Build history of the part. All positions in model axes, mm. A direction names the side the tool comes from. Round coordinates to 2 decimals unless told otherwise and drop trailing zeros. Write each loop counter-clockwise with the first axis right and the second up, starting at its lowest first coordinate (ties: lowest second). Pieces come first, ordered by that corner, then holes. Notation, with made-up numbers: (52, 9) - (92, 9) arc R37 ccw to (92, 47) - close; hole circle Ø3 at (-38, 4.5). An arc over 180 degrees is marked (long way). Write each question's results on one line, items separated by ' | '.
from build123d import *

# Parameters (mm, degrees)
SKETCH1_W           = 35
SKETCH1_H           = 37
SKETCH1_R           = 1.6
BOSS_EXTRUDE1_DEPTH = 3
SKETCH2_W           = 50
SKETCH2_H           = 40
SKETCH2_R           = 1.6
BOSS_EXTRUDE2_DEPTH = 3
FILLET1_R           = 3
FILLET2_R           = 1
FILLET3_R           = 1


with BuildPart() as part:
    # Sketch1 → Boss-Extrude1 (new body)
    with BuildSketch(Plane(origin=(0, 0, 0), x_dir=(1, 0, 0), z_dir=(0, 1, 0))):
        with Locations((2.595206121, -4.992767018)):
            Rectangle(SKETCH1_W, SKETCH1_H)
        with Locations((-11.904793879, 10.507232982)):
            Circle(SKETCH1_R, mode=Mode.SUBTRACT)
        with Locations((-11.904793879, -17.492767018)):
            Circle(SKETCH1_R, mode=Mode.SUBTRACT)
        with Locations((17.095206121, -17.492767018)):
            Circle(SKETCH1_R, mode=Mode.SUBTRACT)
        with Locations((17.095206121, 10.507232982)):
            Circle(SKETCH1_R, mode=Mode.SUBTRACT)
    extrude(amount=BOSS_EXTRUDE1_DEPTH)

    # Sketch2 → Boss-Extrude2 (add)
    with BuildSketch(Plane.XY.offset(23.492767018)):
        with Locations((2.595206121, -17)):
            Rectangle(SKETCH2_W, SKETCH2_H)
        with Locations((23.595206121, -32)):
            Circle(SKETCH2_R, mode=Mode.SUBTRACT)
        with Locations((23.595206121, -2)):
            Circle(SKETCH2_R, mode=Mode.SUBTRACT)
        with Locations((-18.404793879, -2)):
            Circle(SKETCH2_R, mode=Mode.SUBTRACT)
        with Locations((-18.404793879, -32)):
            Circle(SKETCH2_R, mode=Mode.SUBTRACT)
    extrude(amount=BOSS_EXTRUDE2_DEPTH)

    # Fillet1
    fillet1_edges = [part.edges().sort_by_distance(p)[0] for p in [
        (2.595206121, 0, 23.492767018),
    ]]
    fillet(fillet1_edges, radius=FILLET1_R)

    # Fillet2
    fillet2_edges = [part.edges().sort_by_distance(p)[0] for p in [
        (-14.904793879, -1.5, 23.492767018),
    ]]
    fillet(fillet2_edges, radius=FILLET2_R)

    # Fillet3
    fillet3_edges = [part.edges().sort_by_distance(p)[0] for p in [
        (20.095206121, -1.5, 23.492767018),
    ]]
    fillet(fillet3_edges, radius=FILLET3_R)


solid = part.part
(1) Slice it at C-C, the plane z = 8.5. Write the cut outline in (x, y), and give its area (3 significant figures).
Worked answers:
outline: (-14.9, 0) - (20.1, 0) - (20.1, 3) - (-14.9, 3) - close | area: 105 mm2
(2) Two-plate mould, pull along X, no slides. Class faces 1 (the cylindrical face through (-17.67, -33.42, 24.97)), 2 (the flat face through (2, -17, 26.493)), 3 (the flat face through (27.595, -17, 25)), 4 (the flat face through (-22.405, -17, 25)): released by +X, released by -X, zero draft, split by the parting line, or undercut.
Worked answers:
face 1: undercut | face 2: zero draft | face 3: released by +X | face 4: released by -X
(3) Slice it at B-B, the plane x = 10.5. Write the cut outline in (y, z), and give its area (3 significant figures).
Worked answers:
outline: (-37, 23.49) - (-3, 23.49) arc R3 cw to (0, 20.49) - (0, -13.51) - (3, -13.51) - (3, 26.49) - (-37, 26.49) - close | area: 233 mm2
(4) Tool access for faces 5 (the flat face through (2, 0, 3)), 6 (the flat face through (20.095, 2, 5)), 7 (the cylindrical face through (-10.38, 1.48, -10.99)), 8 (the flat face through (2, 3, 6)), 9 (the flat face through (-14.905, 2, 5)): list every direction of +Z, -Z, +X, -X, +Y, -Y with a clear straight run to the whole face (end or side of a thin tool).
Worked answers:
face 5: -Z, +X, -X, -Y | face 6: -Z, +X, +Y, -Y | face 7: +Y, -Y | face 8: +Z, -Z, +X, -X, +Y | face 9: -Z, -X, +Y, -Y
(5) Slice it at A-A, the plane y = -32. Write the cut outline in (x, z).
Worked answers:
outline: (-22.4, 23.49) - (-20, 23.49) - (-20, 26.49) - (-22.4, 26.49) - close; (-16.8, 23.49) - (22, 23.49) - (22, 26.49) - (-16.8, 26.49) - close; (25.2, 23.49) - (27.6, 23.49) - (27.6, 26.49) - (25.2, 26.49) - close
(6) Slice it at D-D, the plane y = -18. Write the cut outline in (x, z).
Worked answers:
outline: (-22.4, 23.49) - (27.6, 23.49) - (27.6, 26.49) - (-22.4, 26.49) - close
(7) Flat gauge pins, fed straight in: pin 1 Ø10 at (x, y) = (-1, -23) entering from -Z; pin 2 Ø8 at (x, z) = (-4.5, -9.5) entering from -Y; pin 3 Ø4 at (y, z) = (0.5, 7) entering from -X. Where does each tip first touch, or does it go through?
Worked answers:
pin 1: stops at z = 23.49 | pin 2: stops at y = 0 | pin 3: stops at x = -14.9
(8) Drill centre lines: probe 1 along Z at (x, y) = (9, -33); probe 2 along Y at (x, z) = (-9.5, -1.5). Where is each one in solid material? Low to high. Write a range as [from, to].
Worked answers:
probe 1: z = [23.49, 26.49] | probe 2: y = [0, 3]
